Geometry check sheet. Reference: the model listing, model coordinates, mm. A direction names the side the tool comes from. Give positions to 0.01 mm unless a question says otherwise; leave off trailing zeros. Loops run counter-clockwise (first coordinate to the right, second up) from the corner with the lowest first, then second, coordinate; pieces in that order, holes last. Notation, with made-up numbers: (62, -8) -> (86, -8) arc R9 cw to (86, 4) -> close; hole circle Ø7 at (-26, 50). An arc over 180 degrees is marked (long way). One line per question, with ' | ' between items.
Autodesk Fusion 360 part; units mm, degrees
sketch "Skizze3" plane through (0, 0, 0) normal (0, 1, 0) x (1, 0, 0)
  line L0 (167.5736, -30) -> (33, -30)
  line L1 (31, -28) -> (31, -14.6863)
  line L2 (31.5858, -13.2721) -> (70.4645, 25.6066)
  line L3 (81.0711, 30) -> (230, 30)
  line L4 (199.3934, -4.3934) -> (178.1802, -25.6066)
  line L5 (210, 0) -> (230, 0)
  circle A0 centre (230, 15) radius 4.5
  circle A1 centre (211.5, 15) radius 2.1
  circle A2 centre (248.5, 15) radius 2.1
  circle A3 centre (248.5, 15) radius 7.5
  circle A4 centre (230, 15) radius 15
  line L6 (236.0811, 1.2879) -> (251.5405, 8.144)
  line L7 (251.3776, 21.926) -> (236.0828, 28.7113)
  arc A5 (167.5736, -30) -> (178.1802, -25.6066) centre (167.5736, -15) ccw
  arc A6 (210, 0) -> (199.3934, -4.3934) centre (210, -15) ccw
  arc A7 (81.0711, 30) -> (70.4645, 25.6066) centre (81.0711, 15) ccw
  arc A8 (31.5858, -13.2721) -> (31, -14.6863) centre (33, -14.6863) ccw
  arc A9 (31, -28) -> (33, -30) centre (33, -28) ccw
  line L8 (89.8088, -15.25) -> (156.3088, -15.25)
  line L9 (89.8088, 15.25) -> (89.8088, -15.25)
  line L10 (156.3088, -15.25) -> (156.3088, 15.25)
  line L11 (156.3088, 15.25) -> (89.8088, 15.25)
  circle A10 centre (160.5588, 9) radius 2.05
  circle A11 centre (85.5588, 9) radius 2.05
  circle A12 centre (85.5588, -9) radius 2.05
  circle A13 centre (160.5588, -9) radius 2.05
  line L12 (171.3088, 12) -> (171.3088, -4.0221)
  line L13 (176.4301, -6.1435) -> (192.4523, 9.8787)
  line L14 (190.331, 15) -> (174.3088, 15)
  arc A14 (174.3088, 15) -> (171.3088, 12) centre (174.3088, 12) ccw
  arc A15 (171.3088, -4.0221) -> (176.4301, -6.1435) centre (174.3088, -4.0221) ccw
  arc A16 (192.4523, 9.8787) -> (190.331, 15) centre (190.331, 12) ccw
  circle A17 centre (49, -20) radius 2.05
  circle A18 centre (69, 10) radius 2.05
  circle A19 centre (69, -20) radius 2.05
  dimension "d66" = 9
  dimension "d68" = 4.2
  dimension "d69" = 18.5
  dimension "d70" = 4.2
  dimension "d71" = 18.5
  dimension "d72" = 15
  dimension "d73" = 15
  dimension "d74" = 30
  dimension "d103" = 15
  dimension "d104" = 15
  dimension "d105" = 15
  dimension "d106" = 2
  dimension "d115" = 230
  dimension "d119" = 31
  dimension "d120" = 135
  dimension "d121" = 2
  dimension "d134" = 15.25
  dimension "d135" = 15.25
  dimension "d136" = 33.25
  dimension "d137" = 33.25
  dimension "d138" = 4.1
  dimension "d139" = 18
  dimension "d140" = 75
  dimension "d143" = 18.2
  dimension "d144" = 15.25
  dimension "d145" = 9
  dimension "d146" = 37.5
  dimension "d147" = 90
  dimension "d148" = 3
  dimension "d149" = 3
  dimension "d150" = 3
  dimension "d169" = 4.1
  dimension "d170" = 10
  dimension "d171" = 30
  dimension "d172" = 10
  dimension "d173" = 18
  dimension "d174" = 20
  dimension "d175" = 60
  dimension "d176" = 135
  dimension "d177" = 15
  dimension "d178" = 15
  dimension "d179" = 20
  dimension "d180" = 15
extrude "Extrusion16" add sketch "Skizze3" along normal blind 10
sketch "Skizze7" plane through (0, 10, 0) normal (0, 1, 0) x (-1, 0, 0)
  circle A0 centre (-248.5, -15) radius 2.1
  circle A1 centre (-85.5588, -9) radius 2.05
  line L0 (-89.8088, -15.25) -> (-156.3088, -15.25)
  line L1 (-156.3088, -15.25) -> (-156.3088, 15.25)
  line L2 (-156.3088, 15.25) -> (-89.8088, 15.25)
  line L3 (-89.8088, 15.25) -> (-89.8088, -15.25)
  circle A2 centre (-160.5588, 9) radius 2.05
  circle A3 centre (-85.5588, 9) radius 2.05
  circle A4 centre (-211.5, -15) radius 2.1
  circle A5 centre (-160.5588, -9) radius 2.05
  circle A6 centre (-230, -15) radius 4.5
  arc A7 (-192.4523, -9.8787) -> (-190.331, -15) centre (-190.331, -12) ccw
  line L4 (-192.4523, -9.8787) -> (-176.4301, 6.1435)
  arc A8 (-171.3088, 4.0221) -> (-176.4301, 6.1435) centre (-174.3088, 4.0221) ccw
  line L5 (-171.3088, 4.0221) -> (-171.3088, -12)
  arc A9 (-174.3088, -15) -> (-171.3088, -12) centre (-174.3088, -12) ccw
  line L6 (-174.3088, -15) -> (-190.331, -15)
  arc A10 (-31.5858, 13.2721) -> (-31, 14.6863) centre (-33, 14.6863) ccw
  line L7 (-31, 14.6863) -> (-31, 28)
  arc A11 (-31, 28) -> (-33, 30) centre (-33, 28) ccw
  line L8 (-33, 30) -> (-167.5736, 30)
  arc A12 (-167.5736, 30) -> (-178.1802, 25.6066) centre (-167.5736, 15) ccw
  line L9 (-178.1802, 25.6066) -> (-199.3934, 4.3934)
  arc A13 (-210, 0) -> (-199.3934, 4.3934) centre (-210, 15) ccw
  line L10 (-210, 0) -> (-230, 0)
  arc A14 (-230, 0) -> (-236.0811, -1.2879) centre (-230, -15) ccw
  line L11 (-236.0811, -1.2879) -> (-251.5405, -8.144)
  arc A15 (-251.5405, -8.144) -> (-251.3776, -21.926) centre (-248.5, -15) ccw
  line L12 (-251.3776, -21.926) -> (-236.0828, -28.7113)
  arc A16 (-236.0828, -28.7113) -> (-230, -30) centre (-230, -15) ccw
  line L13 (-230, -30) -> (-81.0711, -30)
  arc A17 (-81.0711, -30) -> (-70.4645, -25.6066) centre (-81.0711, -15) ccw
  line L14 (-70.4645, -25.6066) -> (-31.5858, 13.2721)
  line L15 (-143.8088, 21) -> (-145.8088, 21)
  line L16 (-146.3088, 21.5) -> (-146.3088, 23.5)
  line L17 (-145.8088, 24) -> (-143.8088, 24)
  line L18 (-143.3088, 23.5) -> (-143.3088, 21.5)
  arc A18 (-146.3088, 21.5) -> (-145.8088, 21) centre (-145.8088, 21.5) ccw
  arc A19 (-143.8088, 21) -> (-143.3088, 21.5) centre (-143.8088, 21.5) ccw
  arc A20 (-143.3088, 23.5) -> (-143.8088, 24) centre (-143.8088, 23.5) ccw
  arc A21 (-145.8088, 24) -> (-146.3088, 23.5) centre (-145.8088, 23.5) ccw
  line L19 (-102.3088, 24) -> (-100.3088, 24)
  arc A22 (-99.8088, 23.5) -> (-100.3088, 24) centre (-100.3088, 23.5) ccw
  arc A23 (-100.3088, 21) -> (-99.8088, 21.5) centre (-100.3088, 21.5) ccw
  line L20 (-100.3088, 21) -> (-102.3088, 21)
  arc A24 (-102.3088, 24) -> (-102.8088, 23.5) centre (-102.3088, 23.5) ccw
  line L21 (-99.8088, 23.5) -> (-99.8088, 21.5)
  arc A25 (-102.8088, 21.5) -> (-102.3088, 21) centre (-102.3088, 21.5) ccw
  line L22 (-102.8088, 21.5) -> (-102.8088, 23.5)
  line L23 (-145.8088, -21) -> (-143.8088, -21)
  arc A26 (-143.3088, -21.5) -> (-143.8088, -21) centre (-143.8088, -21.5) ccw
  arc A27 (-143.8088, -24) -> (-143.3088, -23.5) centre (-143.8088, -23.5) ccw
  line L24 (-143.8088, -24) -> (-145.8088, -24)
  arc A28 (-145.8088, -21) -> (-146.3088, -21.5) centre (-145.8088, -21.5) ccw
  line L25 (-143.3088, -21.5) -> (-143.3088, -23.5)
  arc A29 (-146.3088, -23.5) -> (-145.8088, -24) centre (-145.8088, -23.5) ccw
  line L26 (-146.3088, -23.5) -> (-146.3088, -21.5)
  circle A30 centre (-49, 20) radius 2.05
  circle A31 centre (-69, -10) radius 2.05
  circle A32 centre (-69, 20) radius 2.05
  dimension "d151" = 3
  dimension "d152" = 3
  dimension "d153" = 6
  dimension "d154" = 0.5
  dimension "d155" = 3
  dimension "d156" = 3
  dimension "d157" = 0.5
  dimension "d158" = 6
  dimension "d159" = 10
  dimension "d160" = 10
  dimension "d163" = 3
  dimension "d164" = 3
  dimension "d165" = 0.5
  dimension "d166" = 6
  dimension "d167" = 10
extrude "Extrusion18" cut sketch "Skizze7" against normal blind 10 contours L15 L16 L17 L18 A18 A19 A20 A21 | L19 A22 A23 L20 A24 L21 A25 L22 | L23 A26 A27 L24 A28 L25 A29 L26
equation "d134 = 15 mm + tolerance"
equation "d135 = 15 mm + tolerance"
equation "d136 = 33 mm + tolerance"
equation "d137 = 33 mm + tolerance"
equation "d144 = 15 mm + tolerance"
equation "tolerance = 0.25 mm"
Item 1: Set-up check for faces 4 (the face through (142, 0, -20)), 5 (the face through (123, 5, 15.25)): record each of +Z, -Z, +X, -X, +Y, -Y from which the full face is reachable in a straight line by a thin tool's end or side.
Result:
face 4: +Z, -Z, +X, -X, -Y | face 5: +Y, -Y
Item 2: Release check for a two-part mould opening along X. For faces 1 (the face through (154, 5, -30)), 2 (the face through (256, 5, -15)), 3 (the face through (83.51, 4.93, 9.09)) record: pulls with the +X half, pulls with the -X half, needs draft (parallel to the pull), parting line crosses it, or undercut.
Result:
face 1: needs draft | face 2: pulls with the +X half | face 3: undercut
Item 3: Sectioned sample at C-C (y = 1.75). Give the number of separate pieces and of enclosed holes in the cut face, plus the area to 3 significant figures.
Result:
separate pieces: 1 | enclosed holes: 15 | area: 7,720 mm2
Item 4: Sectioned sample at B-B (x = 49). Record the cut outline in (y, z).
Result:
outline: (0, -4.14) -> (10, -4.14) -> (10, 17.95) -> (0, 17.95) -> close; (0, 22.05) -> (10, 22.05) -> (10, 30) -> (0, 30) -> close
Item 5: Sectioned sample at A-A (x = 137). Record the cut outline in (y, z).
Result:
outline: (0, -30) -> (10, -30) -> (10, -15.25) -> (0, -15.25) -> close; (0, 15.25) -> (10, 15.25) -> (10, 30) -> (0, 30) -> close
Item 6: Depth check by flat-ended pin: pin 1 Ø4 at (y, z) = (7.5, -8.5) entering from -X; pin 2 Ø1.6 at (y, z) = (4, -22.5) entering from +X; pin 3 Ø5 at (x, y) = (225.5, 5.5) entering from +Z. Enter the tip coordinate at first touch or a pass-through.
Result:
pin 1: x = 51.36 | pin 2: x = 251.87 | pin 3: z = 0
Item 7: Scan lines: probe 1 along X at (y, z) = (2.25, 9); probe 2 along X at (y, z) = (2.5, 20); probe 3 along X at (y, z) = (2, 19). Record each from-to range of solid material in increasing order.
Result:
probe 1: 35.86 to 83.51, 87.61 to 89.81, 156.31 to 158.51, 162.61 to 194.79 | probe 2: 31 to 46.95, 51.05 to 66.95, 71.05 to 183.79 | probe 3: 31 to 47.21, 50.79 to 67.21, 70.79 to 184.79
